Source: CAD feature listing. Evaluate the final solid. Frame: model axes, mm. Round coordinates to 2 decimals unless told otherwise and drop trailing zeros. Order: outer loops, then holes, each group sorted by start corner. A loop starts at its lowest first (then second) coordinate and runs counter-clockwise, first axis right, second up. Notation, with made-up numbers: (85, -20.5) - (139, -20.5) arc R5 ccw to (139, -15.5) - close; hole circle Ø5 at (49.5, -0.75). An arc over 180 degrees is marked (long way). Return JSON: item names as keys, results as strings. Group by question number.
1) Ray query, line 1 (X direction, y = -25, z = 127.5); line 2 (X direction, y = 202, z = 20); line 3 (X direction, y = 14.5, z = -3.5). Return the intervals inside material, ascending. Write a range as from..to.
2) Section B-B, the plane y = 199.5. Return loops of the section in (x, z), plus the area to 3 significant figures.
3) Section D-D, the plane z = 308. Return loops of the section in (x, y), plus the area to 3 significant figures.
4) Section C-C, the plane x = -1099.5. Return loops of the section in (y, z).
5) Section A-A, the plane z = 0. Return loops of the section in (x, y), plus the area to 3 significant figures.
6) Contact query for flat-ended pins moving along their axis: P1, Ø10, axis at y = 89.5, z = -263, coming from the -X side; P2, Ø1, axis at y = 103, z = -268.5, coming from the -X side; P3, Ø1.5, axis at x = -300, z = -158.5, coming from the -Y side. Output: stop coordinate, or through.
```python
from build123d import *

# Parameters (mm, degrees)
SKETCH3_R                = 150
BOSS_EXTRUDE1_DEPTH      = 650
BOSS_EXTRUDE1_DEPTH_BACK = 1800
SCALE1_SCALE             = 0.5


with BuildPart() as part:
    # Sketch1 → Revolve1 (revolve)
    with BuildSketch(Plane.XY):
        with BuildLine():
            Line((0, 0), (1501.072590683, 0))
            ThreePointArc((1501.072590683, 0), (750.536295342, 750.536295342), (0, 0))
        make_face()
    revolve(axis=Axis((0, 0, 0), (1, 0, 0)))

    # Sketch3 → Boss-Extrude1 (add, two sides)
    with BuildSketch(Plane(origin=(0, 0, 0), x_dir=(0, 0, -1), z_dir=(1, 0, 0))) as boss_extrude1_sk:
        Circle(SKETCH3_R)
    extrude(amount=BOSS_EXTRUDE1_DEPTH)
    extrude(boss_extrude1_sk.sketch, amount=-BOSS_EXTRUDE1_DEPTH_BACK)

    # Sketch4 → Revolve2 (revolve)
    with BuildSketch(Plane.XY):
        with BuildLine():
            Line((-1710.603610822, 0), (-3210.603610822, 0))
            ThreePointArc((-3210.603610822, 0), (-2460.603610822, 750), (-1710.603610822, 0))
        make_face()
    revolve(axis=Axis((-1710.603610822, 0, 0), (-1, 0, 0)))


with BuildPart() as part_1:
    # Scale1: scaled about (-853.378556816, 0, 0)
    add(part.part.scale(SCALE1_SCALE).moved(Location((-426.689278408, 0, 0))))


solid = part_1.part
```
Geometry check:
{
 "1": {"line 1": "-2008.76..-1305.22, -403.48..300.64", "line 2": "-1972.3..-1341.68, -367.05..264.21", "line 3": "-2031.69..323.55"},
 "2": {"outline": "circle Ø635.06 at (-1656.99, 0); circle Ø635.69 at (-51.42, 0)", "area": "634,000 mm2"},
 "3": {"outline": "circle Ø427.84 at (-1656.99, 0); circle Ø428.78 at (-51.42, 0)", "area": "288,000 mm2"},
 "4": {"outline": "circle Ø150 at (0, 0)"},
 "5": {"outline": "(-1289.57, -75) - (-419.12, -75) arc R375.27 ccw (long way) to (-419.12, 75) - (-1289.57, 75) arc R375 ccw (long way) to start", "area": "1,010,000 mm2"},
 "6": {"P1": "x = -1914.28", "P2": "x = -1898.26", "P3": "y = -233.14"}
}
